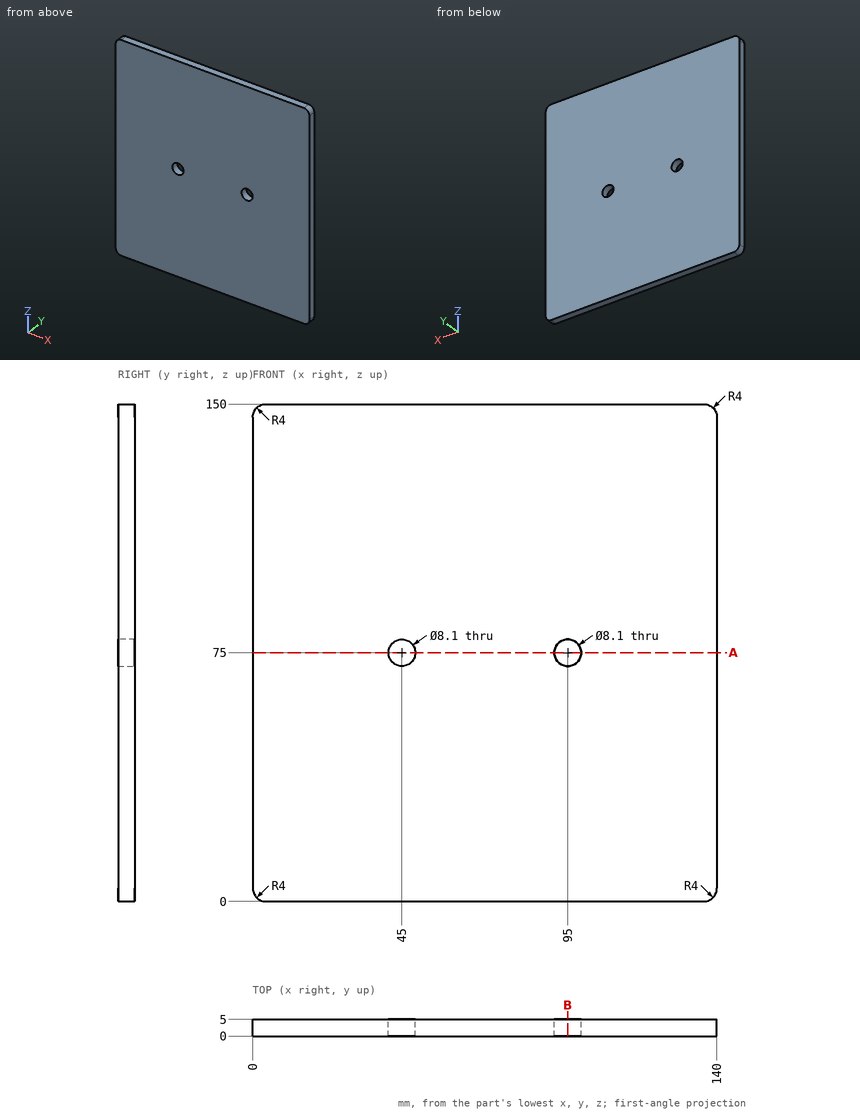
The drawing under review shows one solid part. Ordinate dimensions are in mm from its lowest x, y, z. Round coordinates to 2 decimals unless told otherwise and drop trailing zeros. Loops run counter-clockwise (first coordinate to the right, second up) from the corner with the lowest first, then second, coordinate; pieces in that order, holes last. Notation, with made-up numbers: (-8.5, -2.5) - (4.5, -2.5) arc R16 ccw to (4.5, 16.5) - close; hole circle Ø9 at (83.5, -7). An arc over 180 degrees is marked (long way). Use a Markdown table: item, result. Add a question column.
Q1. Add section B-B (x = 95). State the section outline as (y, z) points.
Q2. Add section A-A (z = 75). State the section outline as (x, y) points, plus the area to 3 significant figures.
Q3. For probe 1 along X at (y, z) = (1.2, 75); probe 2 along Z at (x, y) = (44, 4.5); probe 3 along Z at (x, y) = (47, 3), list the stretches that pass through material, from the lowest coordinate up.
Worked answers:
| question | item | result |
|---|---|---|
| 1 | outline | (0, 0) - (5, 0) - (5, 70.95) - (0, 70.95) - close; (0, 79.05) - (5, 79.05) - (5, 150) - (0, 150) - close |
| 2 | outline | (0, 0) - (40.95, 0) - (40.95, 5) - (0, 5) - close; (49.05, 0) - (90.95, 0) - (90.95, 5) - (49.05, 5) - close; (99.05, 0) - (140, 0) - (140, 5) - (99.05, 5) - close |
| 2 | area | 619 mm² |
| 3 | probe 1 | 0 to 40.95, 49.05 to 90.95, 99.05 to 140 |
| 3 | probe 2 | 0 to 71.08, 78.92 to 150 |
| 3 | probe 3 | 0 to 71.48, 78.52 to 150 |
